The listing builds one solid part. Answer for the finished solid, in the listing's coordinates (mm). A direction names the side the tool comes from. Coordinates: 2 decimals unless noted, no trailing zeros. Order: outer loops, then holes, each group sorted by start corner. A loop starts at its lowest first (then second) coordinate and runs counter-clockwise, first axis right, second up.
from build123d import *

# Parameters (mm, degrees)
F0_W     = 1
F0_H     = 1
F1_DEPTH = 8.9


with BuildPart() as f1:
    # F0 (on Top) → F1 (new body)
    with BuildSketch(Plane.XY):
        with Locations((-11, 0.5)):
            Rectangle(F0_W, F0_H)
        with BuildLine():
            Line((-14.5, 10), (-14.5, 0))
            Line((-14.5, 0), (-11.5, 0))
            Line((-11.5, 0), (-11.5, 1))
            Line((-11.5, 1), (-11.5, 8))
            ThreePointArc((-11.5, 8), (-10.914214, 9.414214), (-9.5, 10))
            Line((-9.5, 10), (-5, 10))
            ThreePointArc((-5, 10), (-3.585786, 9.414214), (-3, 8))
            Line((-3, 8), (-3, 1))
            Line((-3, 1), (-3, 0))
            Line((-3, 0), (0, 0))
            Line((0, 0), (0, 10))
            ThreePointArc((0, 10), (-0.87868, 12.12132), (-3, 13))
            Line((-3, 13), (-11.5, 13))
            ThreePointArc((-11.5, 13), (-13.62132, 12.12132), (-14.5, 10))
        make_face()
        with Locations((-3.5, 0.5)):
            Rectangle(F0_W, F0_H)
    extrude(amount=F1_DEPTH)


solid = f1.part
(1) Find section C-C on z = 5.5. Determine the outline of the cut face in (x, y), then the cut area to 3 significant figures.
(2) Find section B-B on x = -10.75. Determine the outline of the cut face in (y, z), then the cut area to 3 significant figures.
(3) Find the intervals of material crossed by probe 1 along X at (y, z) = (3, 3.5); probe 2 along X at (y, z) = (8.5, 6.25); probe 3 along Y at (x, z) = (-5.5, 4.5), in increasing order.
(4) The mould has two halves that part along X. Classify faces 4 (the flat face through (-2, 0, 4)), 5 (the flat face through (-3.5, 1, 4.4)), 6 (the cylindrical face through (-0.86, 12.1, 4.39)): pulls with the +X half, pulls with the -X half, needs draft (parallel to the pull), parting line crosses it, or undercut.
(5) Find section D-D on x = -9.25. Determine the outline of the cut face in (y, z), then the cut area to 3 significant figures.
(6) A tool of negligible diameter and unlimited length cuts with its end or side. For faces 1 (the cylindrical face through (-3.6, 9.43, 4.39)), 2 (the flat face through (-4, 0.5, 4.4)), 3 (the flat face through (-7, 11, 0)), from which of +Z, -Z, +X, -X, +Y, -Y can it reach the whole face along a straight path? Write none if from no direction.
(7) Find section A-A on y = 1.25. Determine the outline of the cut face in (x, z), then the cut area to 3 significant figures.
(8) Given pin 1 Ø1 at (x, z) = (-12.5, 6) entering from -Y; pin 2 Ø3.5 at (x, z) = (-8, 4.5) entering from -Y; pin 3 Ø5 at (x, y) = (-8, 2.5) entering from -Z; pin 4 Ø1 at (x, z) = (-12.5, 1) entering from +Y, each flat-ended and moving along its own axis, determine where each tip first touches the part or whether it passes through.
Resolved:
1. outline: (-14.5, 0) - (-10.5, 0) - (-10.5, 1) - (-11.5, 1) - (-11.5, 8) arc R2 cw to (-9.5, 10) - (-5, 10) arc R2 cw to (-3, 8) - (-3, 1) - (-4, 1) - (-4, 0) - (0, 0) - (0, 10) arc R3 ccw to (-3, 13) - (-11.5, 13) arc R3 ccw to (-14.5, 10) - close
1. area: 103 mm2
2. outline: (0, 0) - (1, 0) - (1, 8.9) - (0, 8.9) - close; (9.56, 0) - (13, 0) - (13, 8.9) - (9.56, 8.9) - close
2. area: 39.5 mm2
3. probe 1: x = -14.5 to -11.5, -3 to 0
3. probe 2: x = -14.5 to -11.44, -3.06 to 0
3. probe 3: y = 10 to 13
4. face 4: needs draft
4. face 5: undercut
4. face 6: pulls with the +X half
5. outline: (10, 0) - (13, 0) - (13, 8.9) - (10, 8.9) - close
5. area: 26.7 mm2
6. face 1: +Z, -Z
6. face 2: +Z, -Z, -Y
6. face 3: -Z, +X, -X, +Y, -Y
7. outline: (-14.5, 0) - (-11.5, 0) - (-11.5, 8.9) - (-14.5, 8.9) - close; (-3, 0) - (0, 0) - (0, 8.9) - (-3, 8.9) - close
7. area: 53.4 mm2
8. pin 1: stops at y = 0
8. pin 2: stops at y = 9.98
8. pin 3: passes through
8. pin 4: stops at y = 12.96
